Geometry check sheet. Reference: the model listing, model coordinates, mm. A direction names the side the tool comes from. Round coordinates to 2 decimals unless told otherwise and drop trailing zeros. Order: outer loops, then holes, each group sorted by start corner. A loop starts at its lowest first (then second) coordinate and runs counter-clockwise, first axis right, second up. Notation, with made-up numbers: (-7, 16.25) - (50, 16.25) arc R18 ccw to (50, 37.25) - close; hole circle Ø4 at (-29.5, 4). An arc over 180 degrees is marked (long way). Answer as CSV lines item,"result". Start each with the question number.
```python
from build123d import *

# Parameters (mm, degrees)
SKETCH1_R           = 6
SKETCH1_R_2         = 4
SKETCH1_R_3         = 2
BOSS_EXTRUDE1_DEPTH = 2
SKETCH3_R           = 0.94375
CUT_EXTRUDE1_DEPTH  = 2
CIRPATTERN1_COUNT   = 12
BOSS_EXTRUDE2_START = -7
SKETCH1_3_R         = 4
SKETCH1_3_R_2       = 2
BOSS_EXTRUDE2_DEPTH = 5


with BuildPart() as part:
    # Sketch1 → Boss-Extrude1 (new, symmetric)
    # profile 1 of 2: a face of its own
    with BuildSketch(Plane.XY):
        Circle(SKETCH1_R)
        Circle(SKETCH1_R_2, mode=Mode.SUBTRACT)
    # profile 2 of 2: a face of its own
    with BuildSketch(Plane.XY):
        Circle(SKETCH1_R_2)
        Circle(SKETCH1_R_3, mode=Mode.SUBTRACT)
    extrude(amount=BOSS_EXTRUDE1_DEPTH, both=True)

    # Sketch3 → Cut-Extrude1 (cut)
    with BuildSketch(Plane(origin=(0, -6, 0), x_dir=(-1, 0, 0), z_dir=(0, -1, 0))):
        with Locations(Location((0, 0, 0), (0, 0, 90))):
            Circle(SKETCH3_R)
    cut_extrude1 = extrude(amount=-CUT_EXTRUDE1_DEPTH, mode=Mode.SUBTRACT)

    # CirPattern1: Cut-Extrude1 ×12 about axis
    cirpattern1_axis = Axis((0, 0, 0), (0, 0, 1))
    for i in range(1, CIRPATTERN1_COUNT):
        add(cut_extrude1.rotate(cirpattern1_axis, i * 360 / CIRPATTERN1_COUNT), mode=Mode.SUBTRACT)

    # Sketch1<3> → Boss-Extrude2 (add)
    with BuildSketch(Plane.XY.offset(BOSS_EXTRUDE2_START)):
        Circle(SKETCH1_3_R)
        Circle(SKETCH1_3_R_2, mode=Mode.SUBTRACT)
    extrude(amount=BOSS_EXTRUDE2_DEPTH)


solid = part.part
```
1. Go/stop test with flat-tipped pins: pin 1 Ø2.5 at (x, y) = (0, 0) entering from +Z; pin 2 Ø1 at (y, z) = (2, -3) entering from -X; pin 3 Ø1.5 at (x, z) = (3.5, -2) entering from -Y; pin 4 Ø1 at (x, z) = (-2, -6) entering from -Y. Record where each tip stops, or that it passes through.
2. Section check C-C on z = -3.5. Record the boundary of the cut face in (x, y), plus the area to 3 significant figures.
3. Draft check along Y on faces 4 (the face through (4.761, 1.782, -0.435)), 5 (the face through (-0.867, -3.905, -4.535)), 6 (the face through (0.921, 5.014, 0.205)). Enter one of: released by +Y, released by -Y, zero draft, split by the parting line, or undercut.
4. Access from +Z, -Z, +X, -X, +Y, -Y to the whole of each face (thin tool, end or side, straight path). Record for faces 1 (the face through (5.014, -0.921, 0.205)), 2 (the face through (-0.921, -5.014, 0.205)), 3 (the face through (2.01, -3.46, 0.01)).
5. Thickness scan on probe 1 along Y at (x, z) = (0, -4); probe 2 along Z at (x, y) = (4.75, -3.25); probe 3 along Z at (x, y) = (2.5, 4.75). Record the ranges inside material, lowest first.
6. Section check D-D on y = 1.5. Count the separate pieces of the cut face and the enclosed holes in it, plus the area to 3 significant figures.
7. Section check A-A on y = 0. Record the boundary of the cut face in (x, z).
Numbers:
1,pin 1,"passes through"
1,pin 2,"stops at x = -3.71"
1,pin 3,"stops at y = -5.33"
1,pin 4,"stops at y = -3.71"
2,outline,"circle Ø8 at (0, 0); hole circle Ø4 at (0, 0)"
2,area,"37.7 mm2"
3,face 4,"undercut"
3,face 5,"split by the parting line"
3,face 6,"zero draft"
4,face 1,"+X"
4,face 2,"-Y"
4,face 3,"none"
5,probe 1,"y = -4 to -2, 2 to 4"
5,probe 2,"z = -2 to -0.84, 0.84 to 2"
5,probe 3,"z = -2 to -0.92, 0.92 to 2"
6,separate pieces,"2"
6,enclosed holes,"2"
6,area,"58.2 mm2"
7,outline,"(-6, -2) - (-4, -2) - (-4, -7) - (-2, -7) - (-2, 2) - (-6, 2) - (-6, 0.94) - (-4, 0.94) - (-4, -0.94) - (-6, -0.94) - close; (2, -7) - (4, -7) - (4, -2) - (6, -2) - (6, -0.94) - (4, -0.94) - (4, 0.94) - (6, 0.94) - (6, 2) - (2, 2) - close"
